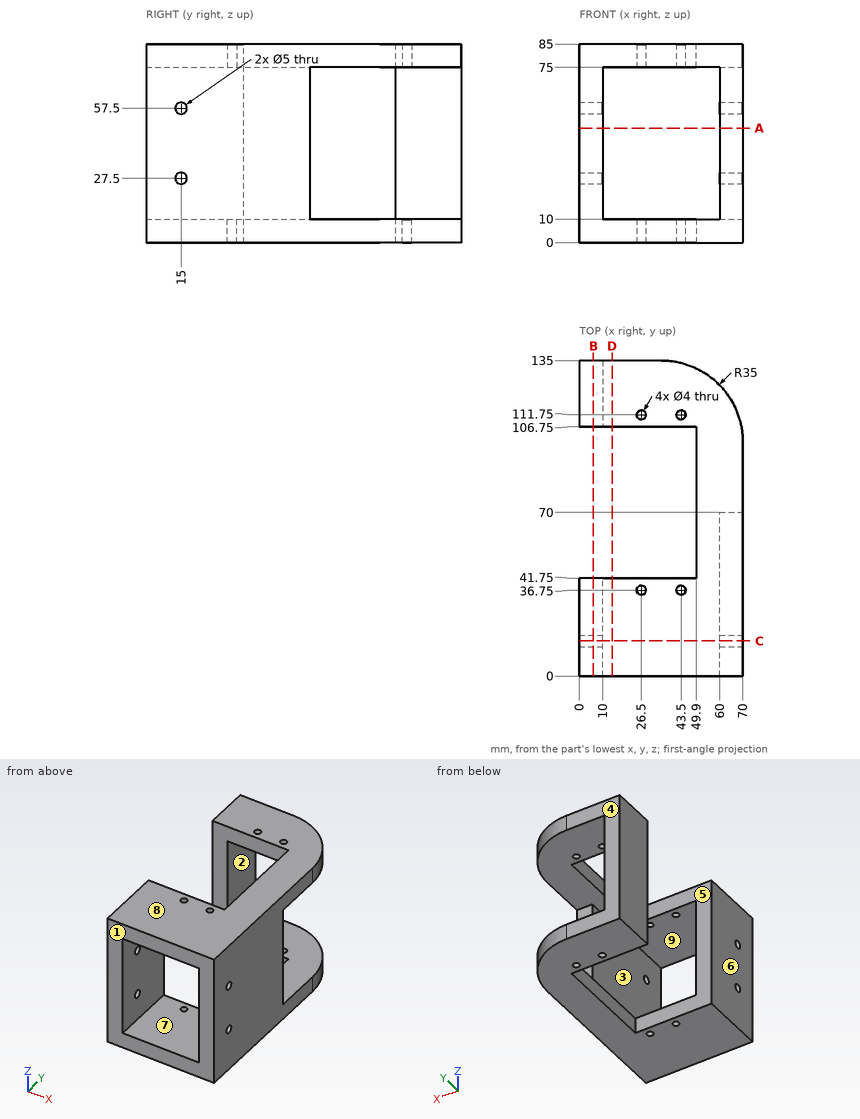
For this review, use the dimensioned drawing (mm, ordinates from the lowest corner) and the shaded views. A direction names the side the tool comes from. Round coordinates to 2 decimals unless told otherwise and drop trailing zeros. Write each loop counter-clockwise with the first axis right and the second up, starting at its lowest first coordinate (ties: lowest second). Pieces come first, ordered by that corner, then holes. Notation, with made-up numbers: (3, 16.5) -> (22, 16.5) arc R26 cw to (22, 40.5) -> close; hole circle Ø3 at (73.25, 26). An arc over 180 degrees is marked (long way). Answer in a Markdown table with one row per item.
Q1. Draft analysis for pull direction Z (two halves, no side actions). For the marked faces 6, 7, 8 and 9, state which applies: +Z half, -Z half, draft (parallel to the pull), parting line (faces both ways), or undercut.
The answers:
| item | result |
|---|---|
| face 6 | draft |
| face 7 | undercut |
| face 8 | +Z half |
| face 9 | undercut |
Q2. Take a section at A-A, the plane z = 49. State the section outline as (x, y) points.
The answers:
| item | result |
|---|---|
| outline | (0, 0) -> (10, 0) -> (10, 41.75) -> (0, 41.75) -> close; (0, 106.75) -> (10, 106.75) -> (10, 135) -> (0, 135) -> close; (60, 0) -> (70, 0) -> (70, 70) -> (60, 70) -> close |
Q3. Take a section at B-B, the plane x = 6. State the section outline as (y, z) points.
The answers:
| item | result |
|---|---|
| outline | (0, 0) -> (41.75, 0) -> (41.75, 85) -> (0, 85) -> close; (106.75, 0) -> (135, 0) -> (135, 85) -> (106.75, 85) -> close; hole circle Ø5 at (15, 27.5); hole circle Ø5 at (15, 57.5) |
Q4. Take a section at D-D, the plane x = 14. State the section outline as (y, z) points.
The answers:
| item | result |
|---|---|
| outline | (0, 0) -> (41.75, 0) -> (41.75, 10) -> (0, 10) -> close; (0, 75) -> (41.75, 75) -> (41.75, 85) -> (0, 85) -> close; (106.75, 0) -> (135, 0) -> (135, 10) -> (106.75, 10) -> close; (106.75, 75) -> (135, 75) -> (135, 85) -> (106.75, 85) -> close |
Q5. For the marked faces 1, 2, 3, 4 and 5, list the 3-axis set-ups (+Z, -Z, +X, -X, +Y, -Y) from which the entire face can be reached by the end or side of a thin tool; tool diameter is ignored.
The answers:
| item | result |
|---|---|
| face 1 | +Z, -Z, +X, -X, -Y |
| face 2 | +X, +Y, -Y |
| face 3 | +Y, -Y |
| face 4 | +Z, -Z, +X, -X, +Y |
| face 5 | +Z, -Z, -X |
Q6. To check wall thickness, follow L1, parallel to Y at x = 26.5, z = 6; L2, parallel to Z at x = 53, y = 25; L3, parallel to Y at x = 43.5, z = 80.5. State the ranges of each line that lie inside material, in increasing order. Write a range as [from, to].
The answers:
| item | result |
|---|---|
| L1 | [0, 34.75], [38.75, 41.75], [106.75, 109.75], [113.75, 135] |
| L2 | [0, 10], [75, 85] |
| L3 | [0, 34.75], [38.75, 41.75], [106.75, 109.75], [113.75, 133.95] |
Q7. Clearance check with flat-ended pins moving along their axes: pin 1 Ø3.5 at (x, y) = (43.5, 36.75) entering from +Z; pin 2 Ø3 at (y, z) = (82.5, 7.5) entering from -X; pin 3 Ø3 at (x, z) = (57.5, 11) entering from +Y; pin 4 Ø4.5 at (x, y) = (26.5, 111.75) entering from +Z. State where each tip first meets the part, or that it passes through.
The answers:
| item | result |
|---|---|
| pin 1 | through |
| pin 2 | x = 49.9 |
| pin 3 | y = 127.71 |
| pin 4 | z = 85 |
Q8. Take a section at C-C, the plane y = 15. State the section outline as (x, z) points.
The answers:
| item | result |
|---|---|
| outline | (0, 0) -> (70, 0) -> (70, 25) -> (60, 25) -> (60, 10) -> (10, 10) -> (10, 25) -> (0, 25) -> close; (0, 30) -> (10, 30) -> (10, 55) -> (0, 55) -> close; (0, 60) -> (10, 60) -> (10, 75) -> (60, 75) -> (60, 60) -> (70, 60) -> (70, 85) -> (0, 85) -> close; (60, 30) -> (70, 30) -> (70, 55) -> (60, 55) -> close |
